The listing builds one solid part. Answer for the finished solid, in the listing's coordinates (mm). A direction names the side the tool comes from. Round coordinates to 2 decimals unless told otherwise and drop trailing zeros. Order: outer loops, then holes, each group sorted by start corner. A loop starts at its lowest first (then second) coordinate and runs counter-clockwise, first axis right, second up. Notation, with made-up numbers: (60.25, 30.5) - (113.25, 30.5) arc R12 cw to (113.25, 39.5) - close; hole circle Ø10 at (54.5, 71.5). An arc over 180 degrees is marked (long way). One line per item, written item: value. Start each with the question number.
1. For a pull along Z with two mould halves and no side action, classify faces 6 (the flat face through (0, 0, -5)), 7 (the flat face through (0, -2, 9.5)), 8 (the flat face through (0, 0, 0)), 9 (the flat face through (0, 0.8, -4)) as released by +Z, released by -Z, zero draft, split by the parting line, or undercut.
2. Section B-B, the plane z = 7 is taken. Give the vertices of the cut face in (x, y), then the cut area to 3 significant figures.
3. Section C-C, the plane x = 0 is taken. Give the vertices of the cut face in (y, z), then the cut area to 3 significant figures.
4. Section D-D, the plane x = -1.9 is taken. Give the vertices of the cut face in (y, z), then the cut area to 3 significant figures.
5. A tool of negligible diameter and unlimited length cuts with its end or side. For faces 1 (the flat face through (0, -1, 4.2)), 2 (the flat face through (0, 0, 5)), 3 (the flat face through (3, -0.3, -0.1)), 4 (the flat face through (0, -1, -9)), 5 (the cylindrical face through (0.07, -1.59, 5.4)), from which of +Z, -Z, +X, -X, +Y, -Y can it reach the whole face along a straight path? Write none if from no direction.
6. Flat-ended cylindrical pins translate along their axes: P1, Ø0.6, axis at x = -0.5, z = 4, coming from the -Y side; P2, Ø0.6, axis at x = 0, z = -3.5, coming from the -Y side; P3, Ø1.9, axis at x = 0, z = 7, coming from the +Y side (1 decimal); P4, Ø3.5, axis at x = -0.5, z = 7.5, coming from the +Y side. Find the tip coordinate at first contact, or state that the pin passes through.
7. Section A-A, the plane y = 0.3 is taken. Give the vertices of the cut face in (x, z).
8. Straight lines are drawn through the part: line 1 (Z direction, x = 1.5, y = -0.4); line 2 (X direction, y = -1.8, z = 7); line 3 (Z direction, x = 0.4, y = 0.5). For each, find the intervals that lie inside material, in ascending order.
from build123d import *

# Parameters (mm, degrees)
BOSS_EXTRUDE4_DEPTH = 3
CUT_EXTRUDE1_REACH  = 12.124
SKETCH5_R           = 1.6


with BuildPart() as part:
    # Sketch4 → Boss-Extrude4 (new, symmetric)
    with BuildSketch(Plane(origin=(0, 0, 0), x_dir=(0, 0, -1), z_dir=(1, 0, 0))):
        Polygon((-5, -1), (-5, 0.8), (-2.6, 0.8), (-2.6, 0), (2.6, 0), (2.6, 0.8), (5, 0.8), (5, -1), (9.5, -1), (9.5, -2.2), (4.2, -2.2), (4.2, 0), (3.4, 0), (3.4, -0.8), (-3.4, -0.8), (-3.4, 0), (-4.2, 0), (-4.2, -2.2), (-9.5, -2.2), (-9.5, -1), align=None)
    extrude(amount=BOSS_EXTRUDE4_DEPTH, both=True)

    # Sketch5 → Cut-Extrude1 (cut, up to next)
    with BuildSketch(Plane(origin=(0, -1, 0), x_dir=(1, 0, 0), z_dir=(0, 1, 0)), mode=Mode.PRIVATE) as cut_extrude1_sk1:
        with Locations(Location((0, -7, 0), (0, 0, 270))):
            Circle(SKETCH5_R)
    cut_extrude1_tool1 = extrude(cut_extrude1_sk1.sketch, amount=-CUT_EXTRUDE1_REACH, mode=Mode.PRIVATE) & part.part
    # Sketch5 → Cut-Extrude1 (cut, up to next)
    with BuildSketch(Plane(origin=(0, -1, 0), x_dir=(1, 0, 0), z_dir=(0, 1, 0)), mode=Mode.PRIVATE) as cut_extrude1_sk2:
        with Locations(Location((0, 7, 0), (0, 0, 270))):
            Circle(SKETCH5_R)
    cut_extrude1_tool2 = extrude(cut_extrude1_sk2.sketch, amount=-CUT_EXTRUDE1_REACH, mode=Mode.PRIVATE) & part.part
    add(cut_extrude1_tool1.solids().sort_by_distance((0, -1, 7))[0], mode=Mode.SUBTRACT)
    add(cut_extrude1_tool2.solids().sort_by_distance((0, -1, -7))[0], mode=Mode.SUBTRACT)


solid = part.part
Answer list:
1. face 6: released by -Z
1. face 7: released by +Z
1. face 8: undercut
1. face 9: zero draft
2. outline: (-3, -2.2) - (-1.6, -2.2) - (-1.6, -1) - (-3, -1) - close; (1.6, -2.2) - (3, -2.2) - (3, -1) - (1.6, -1) - close
2. area: 3.36 mm²
3. outline: (-2.2, -9.5) - (-1, -9.5) - (-1, -8.6) - (-2.2, -8.6) - close; (-2.2, -5.4) - (-1, -5.4) - (-1, -5) - (0.8, -5) - (0.8, -2.6) - (0, -2.6) - (0, 2.6) - (0.8, 2.6) - (0.8, 5) - (-1, 5) - (-1, 5.4) - (-2.2, 5.4) - (-2.2, 4.2) - (0, 4.2) - (0, 3.4) - (-0.8, 3.4) - (-0.8, -3.4) - (0, -3.4) - (0, -4.2) - (-2.2, -4.2) - close; (-2.2, 8.6) - (-1, 8.6) - (-1, 9.5) - (-2.2, 9.5) - close
3. area: 15.9 mm²
4. outline: (-2.2, -9.5) - (-1, -9.5) - (-1, -5) - (0.8, -5) - (0.8, -2.6) - (0, -2.6) - (0, 2.6) - (0.8, 2.6) - (0.8, 5) - (-1, 5) - (-1, 9.5) - (-2.2, 9.5) - (-2.2, 4.2) - (0, 4.2) - (0, 3.4) - (-0.8, 3.4) - (-0.8, -3.4) - (0, -3.4) - (0, -4.2) - (-2.2, -4.2) - close
4. area: 23.6 mm²
5. face 1: +X, -X, -Y
5. face 2: +Z, +X, -X, +Y
5. face 3: +Z, -Z, +X, +Y, -Y
5. face 4: -Z, +X, -X, +Y
5. face 5: +Y, -Y
6. P1: stops at y = -2.2
6. P2: stops at y = -0.8
6. P3: passes through
6. P4: stops at y = -1
7. outline: (-3, -5) - (3, -5) - (3, -2.6) - (-3, -2.6) - close; (-3, 2.6) - (3, 2.6) - (3, 5) - (-3, 5) - close
8. line 1: z = -5 to -4.2, -3.4 to 3.4, 4.2 to 5
8. line 2: x = -3 to -1.6, 1.6 to 3
8. line 3: z = -5 to -2.6, 2.6 to 5
